Read the model definition and answer for the solid it produces. Units are mm, in the model's axes. A direction names the side the tool comes from. Give positions to 0.01 mm unless a question says otherwise; leave off trailing zeros. Order: outer loops, then holes, each group sorted by start corner. A loop starts at its lowest first (then second) coordinate and runs counter-clockwise, first axis right, second up.
```python
from build123d import *

# Parameters (mm, degrees)
ESQUISSE1_R                  = 11
ESQUISSE1_R_2                = 3.5
BOSS_EXTRU_1_DEPTH           = 21
ESQUISSE3_R                  = 28.5
ESQUISSE3_R_2                = 9.55
ENL_V_MAT_EXTRU_1_DEPTH      = 15
BOSS_EXTRU_2_DEPTH           = 15
R_P_TITION_CIRCULAIRE1_COUNT = 12
BOSS_EXTRUDE1_START          = 10.5
ESQUISSE1_3_R                = 3.5
ESQUISSE1_3_W                = 5
ESQUISSE1_3_H                = 3
BOSS_EXTRUDE1_DEPTH          = 7.5


with BuildPart() as part:
    # Esquisse1 → Boss.-Extru.1 (new body)
    with BuildSketch(Plane.XY):
        Circle(ESQUISSE1_R)
        Circle(ESQUISSE1_R_2, mode=Mode.SUBTRACT)
    extrude(amount=BOSS_EXTRU_1_DEPTH)

    # Esquisse3 → Enlèv. mat.-Extru.1 (cut)
    with BuildSketch(Plane(origin=(0, 0, 3), x_dir=(-1, 0, 0), z_dir=(0, 0, -1))):
        Circle(ESQUISSE3_R)
        Circle(ESQUISSE3_R_2, mode=Mode.SUBTRACT)
    extrude(amount=-ENL_V_MAT_EXTRU_1_DEPTH, mode=Mode.SUBTRACT)

    # Esquisse5 → Boss.-Extru.2 (add)
    with BuildSketch(Plane.XY.offset(3)):
        with BuildLine():
            Line((-1.740349268, 9.390084367), (-1.515334698, 10.782166631))
            Line((-1.515334698, 10.782166631), (1.515334698, 10.782166631))
            Line((1.515334698, 10.782166631), (1.740349268, 9.390084367))
            ThreePointArc((1.740349268, 9.390084367), (0, 9.55), (-1.740349268, 9.390084367))
        make_face()
    boss_extru_2 = extrude(amount=BOSS_EXTRU_2_DEPTH)

    # Répétition circulaire1: Boss.-Extru.2 ×12 about axis
    r_p_tition_circulaire1_axis = Axis((0, 0, 0), (0, 0, 1))
    for i in range(1, R_P_TITION_CIRCULAIRE1_COUNT):
        add(boss_extru_2.rotate(r_p_tition_circulaire1_axis, i * 360 / R_P_TITION_CIRCULAIRE1_COUNT))

    # Esquisse1<3> → Boss-Extrude1 (add, symmetric)
    with BuildSketch(Plane.XY.offset(BOSS_EXTRUDE1_START)):
        Circle(ESQUISSE1_3_R)
        Rectangle(ESQUISSE1_3_W, ESQUISSE1_3_H, mode=Mode.SUBTRACT)
    extrude(amount=BOSS_EXTRUDE1_DEPTH, both=True)


solid = part.part
```
1) The part is cut by section B-B on x = 0. Determine the outline of the cut face in (y, z).
Final values:
outline: (-11, 0) - (-3.5, 0) - (-3.5, 3) - (-1.5, 3) - (-1.5, 18) - (-3.5, 18) - (-3.5, 21) - (-11, 21) - (-11, 18) - (-10.78, 18) - (-10.78, 3) - (-11, 3) - close; (1.5, 3) - (3.5, 3) - (3.5, 0) - (11, 0) - (11, 3) - (10.78, 3) - (10.78, 18) - (11, 18) - (11, 21) - (3.5, 21) - (3.5, 18) - (1.5, 18) - close
2) Consider L1, parallel to Y at x = 0, z = 18.7; L2, parallel to Y at x = -0.5, z = 6; L3, parallel to X at y = 9.5, z = 17.75. Determine where each line is inside the solid, lowest interval first.
Final values:
L1: y = -11 to -3.5, 3.5 to 11
L2: y = -10.78 to -1.5, 1.5 to 10.78
L3: x = -5.11 to -3.59, -1.72 to 1.72, 3.59 to 5.11
3) Given pin 1 (1.5 mm diameter, centred on y = 0.5, z = 11, fed in from -X); pin 2 (3 mm diameter, centred on y = 6.5, z = 5.5, fed in from -X); pin 3 (5 mm diameter, centred on x = -6.5, z = 7.5, fed in from +Y), each flat-ended and moving along its own axis, determine where each tip first touches the part or whether it passes through.
Final values:
pin 1: stops at x = -10.78
pin 2: stops at x = -9.56
pin 3: stops at y = 10.1
4) A tool of negligible diameter and unlimited length cuts with its end or side. For faces 1 (the face through (9.227, -2.462, 10.395)), 2 (the face through (0, -10.782, 10)), 3 (the face through (-9.327, -5.409, 10.395)), 4 (the face through (9.35, -5.37, 10.4)), 5 (the face through (1.63, -10.08, 10.4)), from which of +Z, -Z, +X, -X, +Y, -Y can it reach the whole face along a straight path? Write none if from no direction.
Final values:
face 1: +X
face 2: +X, -X, -Y
face 3: -X, -Y
face 4: +X, -Y
face 5: -Y
5) For a pull along Y with two mould halves and no side action, classify faces 6 (the face through (-2.482, 9.222, 10.395)), 7 (the face through (9.222, 2.482, 10.395)), 8 (the face through (-2.462, -9.227, 10.395)) as released by +Y, released by -Y, zero draft, split by the parting line, or undercut.
Final values:
face 6: released by +Y
face 7: undercut
face 8: released by -Y
6) The part is cut by section A-A on y = 0. Determine the outline of the cut face in (x, z).
Final values:
outline: (-11, 0) - (-3.5, 0) - (-3.5, 3) - (-2.5, 3) - (-2.5, 18) - (-3.5, 18) - (-3.5, 21) - (-11, 21) - (-11, 18) - (-10.78, 18) - (-10.78, 3) - (-11, 3) - close; (2.5, 3) - (3.5, 3) - (3.5, 0) - (11, 0) - (11, 3) - (10.78, 3) - (10.78, 18) - (11, 18) - (11, 21) - (3.5, 21) - (3.5, 18) - (2.5, 18) - close
7) The part is cut by section C-C on z = 2.5. Determine the outline of the cut face in (x, y), and give its area (3 significant figures).
Final values:
outline: circle Ø22 at (0, 0); hole circle Ø7 at (0, 0)
area: 342 mm2
8) The part is cut by section D-D on x = -4.5. Determine the outline of the cut face in (y, z), and give its area (3 significant figures).
Final values:
outline: (-10.04, 0) - (10.04, 0) - (10.04, 3) - (9.85, 3) - (9.85, 18) - (10.04, 18) - (10.04, 21) - (-10.04, 21) - (-10.04, 18) - (-9.85, 18) - (-9.85, 3) - (-10.04, 3) - close
area: 416 mm2
